The listing builds one solid part. Answer for the finished solid, in the listing's coordinates (mm). A direction names the side the tool comes from. Round coordinates to 2 decimals unless told otherwise and drop trailing zeros. Order: outer loops, then holes, each group sorted by start corner. A loop starts at its lowest first (then second) coordinate and runs counter-clockwise, first axis right, second up. Notation, with made-up numbers: (27.5, -7) -> (82.5, -7) arc R27 cw to (82.5, 25) -> close; hole circle Ø9 at (-34, -10.75). An arc over 180 degrees is marked (long way). Return JSON: item names as keys, results as strings. Group by question number.
(1) The part is cut by section D-D (x = 10). Determine the outline of the cut face in (y, z).
(2) Consider line 1 (Y direction, x = 43.1, z = 0); line 2 (Y direction, x = 12.5, z = 0); line 3 (X direction, y = 4.7, z = 0). Determine where each line is inside the solid, lowest interval first. Write a range as [from, to].
(3) Which of the six approach directions +Z, -Z, +X, -X, +Y, -Y give full straight-line access (tool end or side, diameter ignored) to faces 4 (the face through (11.268, 3.666, -1.52)), 5 (the face through (34.432, 5.672, 0.122)), 6 (the face through (42, -3.531, 0)), 7 (the face through (4.703, 0.519, 5.696)), 8 (the face through (42.431, 6.324, 0.039))?
(4) Determine the mould class of faces 1 (the face through (17.093, -5.798, 0.054)), 2 (the face through (42, 3.531, 0)), 3 (the face through (26.17, 7.27, -3.02)) for opening direction Y: +Y half, -Y half, draft (parallel to the pull), parting line (faces both ways), or undercut.
(5) Each of these flat-tipped pins is pushed along its axis until it touches: pin 1 (3 mm diameter, centred on x = 41, z = -3, fed in from -Y); pin 2 (2 mm diameter, centred on x = 15.875, z = 0, fed in from -Y); pin 3 (1 mm diameter, centred on y = -1, z = -1, fed in from +X); pin 4 (4 mm diameter, centred on x = 26.5, z = -2.5, fed in from -Y). Where does it stop, or does it pass through?
(6) The part is cut by section B-B (z = 5). Determine the outline of the cut face in (x, y).
(7) The part is cut by section A-A (x = 50). Determine the outline of the cut face in (y, z), plus the area to 3 significant figures.
(8) The part is cut by section C-C (y = -5). Determine the outline of the cut face in (x, z) (3 decimals), plus the area to 3 significant figures.
from build123d import *

# Parameters (mm, degrees)
F0_R      = 7.874
F1_DEPTH  = 53.086
F3_DEPTH  = 12.7
F6_D      = 3.4544
F6_DEPTH  = 7.71525
F6_START  = 4.2557702
F6_TIP    = 1.0378064612
F8_D      = 7.9375
F8_DEPTH  = 22.225
F8_TIP    = 2.3846655818
F9_R      = 2.7813
F10_DEPTH = 12.7
F13_D     = 2.4384
F15_D     = 2.1844
F15_DEPTH = 7.874
F15_TIP   = 0.6562599681
F16_D     = 1.778
F16_DEPTH = 10.16
F16_START = 7.9960949
F16_TIP   = 0.5341650903


with BuildPart() as f1:
    # F0 (on Right) → F1 (new body)
    with BuildSketch(Plane.YZ):
        Circle(F0_R)
    extrude(amount=F1_DEPTH)

    # F2 (on Top) → F3 (cut, symmetric)
    with BuildSketch(Plane.XY):
        with BuildLine():
            ThreePointArc((31.2166, 3.5306), (27.686, 0), (31.2166, -3.5306))
            Line((31.2166, -3.5306), (67.7581354976, -3.5306))
            Line((67.7581354976, -3.5306), (67.7581354976, 3.5306))
            Line((67.7581354976, 3.5306), (31.2166, 3.5306))
        make_face()
    extrude(amount=F3_DEPTH, both=True, mode=Mode.SUBTRACT)

    # F6
    # its depths count from where the whole tool has entered the part; down to there all is cleared
    with Locations(Plane.XY.offset(11.938).offset(-F6_START)):
        with Locations((6.35, 0)):
            Hole(F6_D / 2, depth=F6_DEPTH)
            with Locations((0, 0, -(F6_DEPTH + F6_TIP / 2))):  # 118° drill point
                Cone(0, F6_D / 2, F6_TIP, mode=Mode.SUBTRACT)

    # F8
    with Locations(Plane(origin=(0, 0, 0), x_dir=(0, -1, 0), z_dir=(-1, 0, 0))):
        with Locations((0, 0)):
            Hole(F8_D / 2, depth=F8_DEPTH)
            with Locations((0, 0, -(F8_DEPTH + F8_TIP / 2))):  # 118° drill point
                Cone(0, F8_D / 2, F8_TIP, mode=Mode.SUBTRACT)

    # F9 (on Front) → F10 (cut, symmetric)
    with BuildSketch(Plane.XZ):
        with Locations((37.211, 0)):
            Circle(F9_R)
    extrude(amount=F10_DEPTH, both=True, mode=Mode.SUBTRACT)

    # F13 (through all)
    with Locations(Plane.XZ.offset(12.7)):
        with Locations((15.875, 0)):
            Hole(F13_D / 2)

    # F15
    with Locations(Plane.YZ.offset(53.086)):
        with Locations((5.4356, 0)):
            Hole(F15_D / 2, depth=F15_DEPTH)
            with Locations((0, 0, -(F15_DEPTH + F15_TIP / 2))):  # 118° drill point
                Cone(0, F15_D / 2, F15_TIP, mode=Mode.SUBTRACT)

    # F16
    # its depths count from where the whole tool has entered the part; down to there all is cleared
    with Locations(Plane.YZ.offset(53.086).offset(-F16_START)):
        with Locations((5.4356, 0)):
            Hole(F16_D / 2, depth=F16_DEPTH)
            with Locations((0, 0, -(F16_DEPTH + F16_TIP / 2))):  # 118° drill point
                Cone(0, F16_D / 2, F16_TIP, mode=Mode.SUBTRACT)


solid = f1.part
Answer below:
{
 "1": {"outline": "circle Ø15.75 at (0, 0); hole circle Ø7.94 at (0, 0)"},
 "2": {"line 1": "y = [-7.87, -3.53], [3.53, 4.55], [6.32, 7.87]", "line 2": "y = [-7.87, -3.97], [3.97, 7.87]", "line 3": "x = [0, 14.66], [17.09, 34.43]"},
 "3": {"face 4": "-X", "face 5": "+Y, -Y", "face 6": "+Z, -Z, +X", "face 7": "+Z", "face 8": "+X"},
 "4": {"face 1": "draft", "face 2": "undercut", "face 3": "parting line"},
 "5": {"pin 1": "stops at y = -7.73", "pin 2": "passes through", "pin 3": "stops at x = 28.02", "pin 4": "stops at y = -7.86"},
 "6": {"outline": "(0, -6.08) -> (53.09, -6.08) -> (53.09, -3.53) -> (31.22, -3.53) arc R3.53 cw to (31.22, 3.53) -> (53.09, 3.53) -> (53.09, 6.08) -> (0, 6.08) -> close; hole circle Ø3.45 at (6.35, 0)"},
 "7": {"outline": "(-3.53, -7.04) -> (-3.53, 7.04) arc R7.87 ccw to start; (3.53, -7.04) arc R7.87 ccw to (3.53, 7.04) -> close; hole circle Ø2.18 at (5.44, 0)", "area": "83.7 mm²"},
 "8": {"outline": "(0, -6.083) -> (53.086, -6.083) -> (53.086, 6.083) -> (0, 6.083) -> close; hole circle Ø2.438 at (15.875, 0); hole circle Ø5.563 at (37.211, 0)", "area": "617 mm²"}
}
